Verification items for the finished model (mm, model axes). A direction names the side the tool comes from. Give positions to 0.01 mm unless a question says otherwise; leave off trailing zeros. Loops run counter-clockwise (first coordinate to the right, second up) from the corner with the lowest first, then second, coordinate; pieces in that order, holes last. Notation, with made-up numbers: (54.25, 41) - (97.25, 41) arc R14 ccw to (97.25, 58) - close; hole circle Ø8 at (12.25, 57.25). An arc over 180 degrees is marked (long way). Use one line per item in the form item = value.
```python
from build123d import *

# Parameters (mm, degrees)
SKETCH_R        = 4
PAD_DEPTH       = 60
SKETCH001_W     = 8
SKETCH001_H     = 20
PAD001_DEPTH    = 25
POCKET_DEPTH    = 8
SKETCH003_R     = 2.5
POCKET001_DEPTH = 30
SKETCH004_R     = 4
SKETCH004_R_2   = 3.7
POCKET002_DEPTH = 55
PAD002_DEPTH    = 8


with BuildPart() as part:
    # Sketch → Pad (new body)
    with BuildSketch(Plane.XY):
        Circle(SKETCH_R)
    extrude(amount=PAD_DEPTH)

    # Sketch001 → Pad001 (new body)
    with BuildSketch(Plane.XY.offset(60)):
        Rectangle(SKETCH001_W, SKETCH001_H)
    extrude(amount=PAD001_DEPTH)

    # Sketch002 → Pocket (cut)
    with BuildSketch(Plane(origin=(-4, 0, 0), x_dir=(0, -1, 0), z_dir=(-1, 0, 0))):
        with BuildLine():
            ThreePointArc((-1.5, 75.769696), (0, 66), (1.5, 75.769696))
            Line((1.5, 85), (1.5, 75.769696))
            Line((1.5, 85), (-1.5, 85))
            Line((-1.5, 85), (-1.5, 75.769696))
        make_face()
    extrude(amount=-POCKET_DEPTH, mode=Mode.SUBTRACT)

    # Sketch003 → Pocket001 (cut)
    with BuildSketch(Plane.XZ.offset(10)):
        with Locations((0, 80.5)):
            Circle(SKETCH003_R)
    extrude(amount=-POCKET001_DEPTH, mode=Mode.SUBTRACT)

    # Sketch004 → Pocket002 (cut)
    with BuildSketch(Plane(origin=(0, 0, 0), x_dir=(1, 0, 0), z_dir=(0, 0, -1))):
        Circle(SKETCH004_R)
        Circle(SKETCH004_R_2, mode=Mode.SUBTRACT)
    extrude(amount=-POCKET002_DEPTH, mode=Mode.SUBTRACT)

    # Sketch005 → Pad002 (new body)
    with BuildSketch(Plane(origin=(-4, 0, 0), x_dir=(0, -1, 0), z_dir=(-1, 0, 0))):
        with BuildLine():
            ThreePointArc((-1.5, 75.348563), (0, 66.4), (1.5, 75.348563))
            Line((1.5, 75.978956), (1.5, 75.348563))
            ThreePointArc((-1.5, 75.978956), (0, 65.8), (1.5, 75.978956))
            Line((-1.5, 75.978956), (-1.5, 75.348563))
        make_face()
    extrude(amount=-PAD002_DEPTH)


solid = part.part
```
1. Depth check by flat-ended pin: pin 1 Ø2 at (y, z) = (6, 20) entering from +X; pin 2 Ø2 at (y, z) = (0.5, 22.5) entering from +X; pin 3 Ø3 at (y, z) = (3, 15.5) entering from +X; pin 4 Ø12 at (y, z) = (7, 19.5) entering from +X. Enter the tip coordinate at first touch or a pass-through.
Result set:
pin_1 = through
pin_2 = 3.7
pin_3 = 3.38
pin_4 = 3.56
2. Section check A-A, the plane z = 71. Record the cut outline in (x, y).
Result set:
outline = (-4, -10) - (4, -10) - (4, -4.6) - (-4, -4.6) - close; (-4, 4.6) - (4, 4.6) - (4, 10) - (-4, 10) - close
3. Section check C-C, the plane y = -5.75. Record the cut outline in (x, z).
Result set:
outline = (-4, 60) - (4, 60) - (4, 85) - (-4, 85) - close; hole circle Ø5 at (0, 80.5)
4. Scan lines: probe 1 along Y at (x, z) = (-2, 76); probe 2 along Y at (x, z) = (1.5, 71); probe 3 along Z at (x, y) = (0, 7.5). Record each from-to range of solid material in increasing order.
Result set:
probe_1 = -10 to -1.5, 1.5 to 10
probe_2 = -10 to -4.6, 4.6 to 10
probe_3 = 60 to 78, 83 to 85
5. Section check B-B, the plane x = 0. Record the cut outline in (y, z), then the cut area to 3 significant figures.
Result set:
outline = (-10, 60) - (-4, 60) - (-4, 55) - (-3.7, 55) - (-3.7, 0) - (3.7, 0) - (3.7, 55) - (4, 55) - (4, 60) - (10, 60) - (10, 78) - (1.5, 78) - (1.5, 75.35) arc R4.6 cw (long way) to (-1.5, 75.35) - (-1.5, 78) - (-10, 78) - close; (-10, 83) - (-1.5, 83) - (-1.5, 85) - (-10, 85) - close; (1.5, 83) - (10, 83) - (10, 85) - (1.5, 85) - close
area = 767 mm²
6. Tool access check on faces 1 (the flat face through (-1, -1.5, 78)), 2 (the cylindrical face through (-0.867, -3.905, 57.465)), 3 (the flat face through (0, 6, 85)). Record the directions out of +Z, -Z, +X, -X, +Y, -Y that give a thin tool (end or side, any length) a straight path to the whole face; none if there is none.
Result set:
face_1 = +Z, +X, -X
face_2 = -Z
face_3 = +Z, +X, -X, +Y, -Y
7. Section check D-D, the plane z = 47. Record the cut outline in (x, y).
Result set:
outline = circle Ø7.4 at (0, 0)
8. Draft check along Z on faces 4 (the cylindrical face through (-0.802, 3.612, 27.115)), 5 (the flat face through (0, -7, 60)), 6 (the cylindrical face through (-0.056, 0.181, 66.404)). Enter one of: released by +Z, released by -Z, zero draft, split by the parting line, or undercut.
Result set:
face_4 = zero draft
face_5 = released by -Z
face_6 = undercut
